```python
from build123d import *

# Parameters (mm, degrees)
F1_DEPTH = 160


with BuildPart() as f1:
    # F0 (on Front) → F1 (new body)
    with BuildSketch(Plane.XZ):
        with BuildLine():
            ThreePointArc((0, 6), (1.757359, 1.757359), (6, 0))
            Line((6, 0), (61, 0))
            Line((61, 0), (116, 0))
            ThreePointArc((116, 0), (120.242641, 1.757359), (122, 6))
            Line((122, 6), (122, 12.8))
            Line((122, 12.8), (120.5, 12.8))
            Line((120.5, 12.8), (120.5, 11.6))
            Line((120.5, 11.6), (117.5, 11.6))
            Line((117.5, 11.6), (117.5, 17.6))
            Line((117.5, 17.6), (120.5, 17.6))
            Line((120.5, 17.6), (120.5, 16.4))
            Line((120.5, 16.4), (122, 16.4))
            Line((122, 16.4), (122, 22.4))
            Line((122, 22.4), (122, 28.4))
            Line((122, 28.4), (120.5, 28.4))
            Line((120.5, 28.4), (120.5, 27.2))
            Line((120.5, 27.2), (117.5, 27.2))
            Line((117.5, 27.2), (117.5, 33.2))
            Line((117.5, 33.2), (120.5, 33.2))
            Line((120.5, 33.2), (120.5, 32))
            Line((120.5, 32), (122, 32))
            Line((122, 32), (122, 38.8))
            ThreePointArc((122, 38.8), (120.242641, 43.042641), (116, 44.8))
            Line((116, 44.8), (61, 44.8))
            Line((61, 44.8), (6, 44.8))
            ThreePointArc((6, 44.8), (1.757359, 43.042641), (0, 38.8))
            Line((0, 38.8), (0, 32))
            Line((0, 32), (1.5, 32))
            Line((1.5, 32), (1.5, 33.2))
            Line((1.5, 33.2), (4.5, 33.2))
            Line((4.5, 33.2), (4.5, 27.2))
            Line((4.5, 27.2), (1.5, 27.2))
            Line((1.5, 27.2), (1.5, 28.4))
            Line((1.5, 28.4), (0, 28.4))
            Line((0, 28.4), (0, 22.4))
            Line((0, 22.4), (0, 16.4))
            Line((0, 16.4), (1.5, 16.4))
            Line((1.5, 16.4), (1.5, 17.6))
            Line((1.5, 17.6), (4.5, 17.6))
            Line((4.5, 17.6), (4.5, 11.6))
            Line((4.5, 11.6), (1.5, 11.6))
            Line((1.5, 11.6), (1.5, 12.8))
            Line((1.5, 12.8), (0, 12.8))
            Line((0, 12.8), (0, 6))
        make_face()
        with BuildLine():
            ThreePointArc((1.9, 38.8), (3.100862, 41.699138), (6, 42.9))
            Line((6, 42.9), (61, 42.9))
            Line((61, 42.9), (116, 42.9))
            ThreePointArc((116, 42.9), (118.899138, 41.699138), (120.1, 38.8))
            Line((120.1, 38.8), (119.45, 38.8))
            Line((119.45, 38.8), (119.45, 38.282159))
            ThreePointArc((119.45, 38.282159), (118.7, 35.7), (117.95, 38.282159))
            Line((117.95, 38.282159), (117.95, 38.8))
            Line((117.95, 38.8), (116, 38.8))
            Line((116, 38.8), (116, 25.9))
            Line((116, 25.9), (118.5, 25.9))
            Line((118.5, 25.9), (118.5, 22.4))
            Line((118.5, 22.4), (118.5, 18.9))
            Line((118.5, 18.9), (116, 18.9))
            Line((116, 18.9), (116, 6))
            Line((116, 6), (117.95, 6))
            Line((117.95, 6), (117.95, 6.517841))
            ThreePointArc((117.95, 6.517841), (118.7, 9.1), (119.45, 6.517841))
            Line((119.45, 6.517841), (119.45, 6))
            Line((119.45, 6), (120.1, 6))
            ThreePointArc((120.1, 6), (118.899138, 3.100862), (116, 1.9))
            Line((116, 1.9), (61, 1.9))
            Line((61, 1.9), (6, 1.9))
            ThreePointArc((6, 1.9), (3.100862, 3.100862), (1.9, 6))
            Line((1.9, 6), (2.55, 6))
            Line((2.55, 6), (2.55, 6.517841))
            ThreePointArc((2.55, 6.517841), (3.3, 9.1), (4.05, 6.517841))
            Line((4.05, 6.517841), (4.05, 6))
            Line((4.05, 6), (6, 6))
            Line((6, 6), (6, 18.9))
            Line((6, 18.9), (3.5, 18.9))
            Line((3.5, 18.9), (3.5, 22.4))
            Line((3.5, 22.4), (3.5, 25.9))
            Line((3.5, 25.9), (6, 25.9))
            Line((6, 25.9), (6, 38.8))
            Line((6, 38.8), (4.05, 38.8))
            Line((4.05, 38.8), (4.05, 38.282159))
            ThreePointArc((4.05, 38.282159), (3.3, 35.7), (2.55, 38.282159))
            Line((2.55, 38.282159), (2.55, 38.8))
            Line((2.55, 38.8), (1.9, 38.8))
        make_face(mode=Mode.SUBTRACT)
    extrude(amount=F1_DEPTH)


solid = f1.part
```
Work out the finished part from the listing and answer in its coordinate system (mm). A direction names the side the tool comes from. Coordinates: 2 decimals unless noted, no trailing zeros. Write each loop counter-clockwise with the first axis right and the second up, starting at its lowest first coordinate (ties: lowest second). Pieces come first, ordered by that corner, then holes.
Q1. Each of these flat-tipped pins is pushed along its axis until it touches: pin 1 Ø1.8 at (y, z) = (-89.5, 14) entering from +X; pin 2 Ø0.8 at (x, y) = (121, -50) entering from +Z; pin 3 Ø3.5 at (x, y) = (118.5, -78) entering from +Z; pin 4 Ø10 at (x, z) = (52, 8.5) entering from -Y. Where does it stop, or does it pass through?
Q2. A cutting plane is placed at B-B, the plane x = 105.5. Give the vertices of the cut face in (y, z).
Q3. Find the intervals of material crossed by line 1 (X direction, y = -11, z = 17); line 2 (X direction, y = -60, z = 37); line 3 (Z direction, x = 46, y = -43), in increasing order.
Q4. A cutting plane is placed at A-A, the plane z = 23. Give the vertices of the cut face in (x, y), then the cut area to 3 significant figures.
Q5. Which of the six approach directions +Z, -Z, +X, -X, +Y, -Y give full straight-line access (tool end or side, diameter ignored) to faces 1 (the face through (0, -79, 22)), 2 (the face through (118.5, -79, 22))?
Findings below:
1. pin 1: stops at x = 117.5
1. pin 2: stops at z = 42.65
1. pin 3: stops at z = 44.75
1. pin 4: passes through
2. outline: (-160, 0) - (0, 0) - (0, 1.9) - (-160, 1.9) - close; (-160, 42.9) - (0, 42.9) - (0, 44.8) - (-160, 44.8) - close
3. line 1: x = 0 to 1.5, 4.5 to 6, 116 to 117.5, 120.5 to 122
3. line 2: x = 0 to 1.9, 4.7 to 6, 116 to 117.3, 120.1 to 122
3. line 3: z = 0 to 1.9, 42.9 to 44.8
4. outline: (0, -160) - (3.5, -160) - (3.5, 0) - (0, 0) - close; (118.5, -160) - (122, -160) - (122, 0) - (118.5, 0) - close
4. area: 1,120 mm2
5. face 1: +Z, -Z, -X, +Y, -Y
5. face 2: +Y, -Y
